Design review of the part built by this model. Coordinates are the model's own, in mm. A direction names the side the tool comes from. Coordinates: 2 decimals unless noted, no trailing zeros. Order: outer loops, then holes, each group sorted by start corner. A loop starts at its lowest first (then second) coordinate and runs counter-clockwise, first axis right, second up. Notation, with made-up numbers: M 10,-1 L 25,-1 A26 cw 25,20 Z; hole C -35,-28 d8. An arc over 180 degrees is marked long. Use CSV: the item, a comma, the result in double quotes.
```python
from build123d import *

# Parameters (mm, degrees)
SKETCH1_R           = 14.2875
BOSS_EXTRUDE1_DEPTH = 12.7
SKETCH2_W           = 48.895
SKETCH2_H           = 6.35
SKETCH2_H_2         = 12.7
BOSS_EXTRUDE2_DEPTH = 144.78
BOSS_EXTRUDE3_START = 12.7
SKETCH3_R           = 14.2875
BOSS_EXTRUDE3_DEPTH = 12.7
SKETCH4_R           = 14.2875
CUT_EXTRUDE1_DEPTH  = 25.654


with BuildPart() as part:
    # Sketch1 → Boss-Extrude1 (new body)
    with BuildSketch(Plane(origin=(0, 0, 0), x_dir=(0, 0, -1), z_dir=(1, 0, 0))):
        with BuildLine():
            Line((-24.4475, 0), (-24.4475, 88.9))
            Line((-24.4475, 88.9), (24.4475, 88.9))
            Line((24.4475, 88.9), (24.4475, 0))
            ThreePointArc((24.4475, 0), (0, -24.4475), (-24.4475, 0))
        make_face()
        Circle(SKETCH1_R, mode=Mode.SUBTRACT)
    extrude(amount=BOSS_EXTRUDE1_DEPTH)

    # Sketch2 → Boss-Extrude2 (add)
    with BuildSketch(Plane.ZY):
        with Locations((0, 33.056893832)):
            Rectangle(SKETCH2_W, SKETCH2_H)
        with Locations((0, 82.55)):
            Rectangle(SKETCH2_W, SKETCH2_H_2)
    extrude(amount=BOSS_EXTRUDE2_DEPTH)

    # Sketch3 → Boss-Extrude3 (add)
    with BuildSketch(Plane.ZY.offset(144.78).offset(BOSS_EXTRUDE3_START)):
        with BuildLine():
            Line((-24.4475, 0), (-24.4475, 88.9))
            Line((-24.4475, 88.9), (24.4475, 88.9))
            Line((24.4475, 88.9), (24.4475, 0))
            ThreePointArc((24.4475, 0), (0, -24.4475), (-24.4475, 0))
        make_face()
        with Locations(Location((0, 0, 0), (0, 0, 180))):
            Circle(SKETCH3_R, mode=Mode.SUBTRACT)
    extrude(amount=-BOSS_EXTRUDE3_DEPTH)

    # Sketch4 → Cut-Extrude1 (cut)
    with BuildSketch(Plane(origin=(0, 88.9, 0), x_dir=(1, 0, 0), z_dir=(0, 1, 0))):
        with Locations(Location((-113.03, 0, 0), (0, 0, 270))):
            Circle(SKETCH4_R)
        with Locations(Location((-72.3392, 0, 0), (0, 0, 270))):
            Circle(SKETCH4_R)
        with Locations(Location((-31.6484, 0, 0), (0, 0, 270))):
            Circle(SKETCH4_R)
    extrude(amount=-CUT_EXTRUDE1_DEPTH, mode=Mode.SUBTRACT)


solid = part.part
```
(1) Add section C-C on x = -52. State the section outline as (y, z) points, and give its area (3 significant figures).
The answers:
outline,"M 29.88,-24.45 L 36.23,-24.45 L 36.23,24.45 L 29.88,24.45 Z; M 76.2,-24.45 L 88.9,-24.45 L 88.9,24.45 L 76.2,24.45 Z"
area,"931 mm2"
(2) Add section B-B on y = 48.5. State the section outline as (x, z) points.
The answers:
outline,"M -157.48,-24.45 L -144.78,-24.45 L -144.78,24.45 L -157.48,24.45 Z; M 0,-24.45 L 12.7,-24.45 L 12.7,24.45 L 0,24.45 Z"
(3) Wall thickness on probe 1 along X at (y, z) = (84.25, 0); probe 2 along Y at (x, z) = (-140, -4.5); probe 3 along Y at (x, z) = (4, 0): over which ranges is each line inside the solid? List them lowest first.
The answers:
probe 1,"x = -157.48 to -127.32, -98.74 to -86.63, -58.05 to -45.94, -17.36 to 12.7"
probe 2,"y = 29.88 to 36.23, 76.2 to 88.9"
probe 3,"y = -24.45 to -14.29, 14.29 to 88.9"
(4) The part is to be moulded in two halves that separate along X. For faces 6 (the face through (6.26, -24.44, -0.54)), 7 (the face through (-157.48, 33, 0)), 8 (the face through (-71, 29.882, 0)), say which applies: pulls with the +X half, pulls with the -X half, needs draft (parallel to the pull), parting line crosses it, or undercut.
The answers:
face 6,"needs draft"
face 7,"pulls with the -X half"
face 8,"undercut"
(5) Add section D-D on x = -113.03. State the section outline as (y, z) points, and give its area (3 significant figures).
The answers:
outline,"M 29.88,-24.45 L 36.23,-24.45 L 36.23,24.45 L 29.88,24.45 Z; M 76.2,-24.45 L 88.9,-24.45 L 88.9,-14.29 L 76.2,-14.29 Z; M 76.2,14.29 L 88.9,14.29 L 88.9,24.45 L 76.2,24.45 Z"
area,"569 mm2"
(6) Clearance check with flat-ended pins moving along their axes: P1, Ø14.5, axis at x = -80.5, z = 10, coming from the -Y side; P2, Ø14.5, axis at y = 2.5, z = 3.5, coming from the +X side; P3, Ø14.5, axis at y = 4.5, z = -11, coming from the -X side; P4, Ø4, axis at x = -33, z = -2.5, coming from the +Y side. State where each tip first meets the part, or that it passes through.
The answers:
P1,"stops at y = 29.88"
P2,"passes through"
P3,"stops at x = -157.48"
P4,"stops at y = 36.23"
(7) For faces 1 (the face through (0, 15, 0)), 2 (the face through (-87, 76.2, 0)), 3 (the face through (-74, 88.9, -17)), 4 (the face through (-151.22, -24.44, 0.54)), 5 (the face through (-86.287, 82.639, -3.097)), list the 3-axis set-ups (+Z, -Z, +X, -X, +Y, -Y) from which the entire face can be reached by the end or side of a thin tool; tool diameter is ignored.
The answers:
face 1,"+Z, -Z, -Y"
face 2,"+Z, -Z"
face 3,"+Z, -Z, +X, -X, +Y"
face 4,"+X, -X, -Y"
face 5,"+Y"
(8) Add section A-A on z = 0. Give the number of separate pieces and of enclosed holes in the cut face, and give its area (3 significant figures).
The answers:
separate pieces,"5"
enclosed holes,"0"
area,"3,820 mm2"
